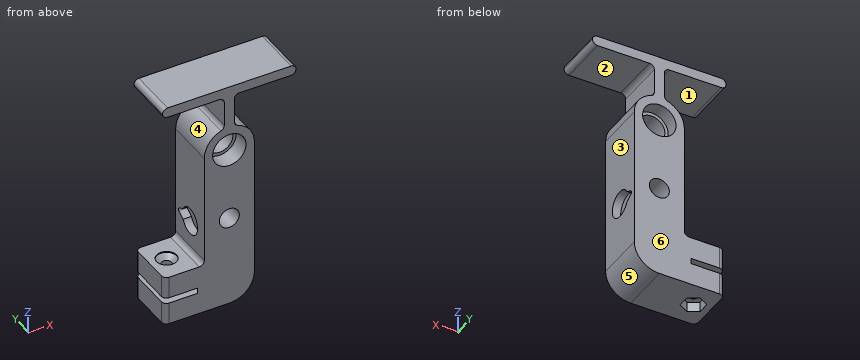
from build123d import *

# Parameters (mm, degrees)
SKETCH1_R           = 4
BOSS_EXTRUDE1_DEPTH = 7.5
SKETCH2_R           = 5
CUT_EXTRUDE1_DEPTH  = 4.1
SKETCH12_R          = 5
SKETCH12_R_2        = 4
CUT_EXTRUDE10_DEPTH = 1
CUT_EXTRUDE3_DEPTH  = 2.5
BOSS_EXTRUDE3_DEPTH = 15
CUT_EXTRUDE7_REACH  = 45.603
SKETCH7_W           = 10
SKETCH7_H           = 1.7
CUT_EXTRUDE8_REACH  = 76.732
SKETCH8_R           = 1.5
CUT_EXTRUDE9_DEPTH  = 3
CUT_EXTRUDE11_DEPTH = 1.7
BOSS_EXTRUDE2_START = -15
BOSS_EXTRUDE2_DEPTH = 15
FILLET8_R           = 1.5
CUT_EXTRUDE12_REACH = 45.829
SKETCH19_R          = 3


with BuildPart() as part:
    # Sketch1 → Boss-Extrude1 (new, symmetric)
    with BuildSketch(Plane(origin=(0, 0, 0), x_dir=(1, 0, 0), z_dir=(0, 1, 0))):
        with BuildLine():
            Line((7.5, 21), (-7.5, 21))
            Line((-7.5, 21), (-7.5, -13.499999984))
            ThreePointArc((-7.5, -13.499999984), (-8e-09, -21), (7.5, -13.5))
            Line((7.5, -13.5), (7.5, 21))
        make_face()
        with Locations(Location((0, -13.5, 0), (0, 0, 270))):
            Circle(SKETCH1_R, mode=Mode.SUBTRACT)
    extrude(amount=BOSS_EXTRUDE1_DEPTH, both=True)

    # Sketch2 → Cut-Extrude1 (cut)
    with BuildSketch(Plane(origin=(0, 7.5, 0), x_dir=(1, 0, 0), z_dir=(0, 1, 0))):
        with Locations(Location((0, -13.5, 0), (0, 0, 270))):
            Circle(SKETCH2_R)
    cut_extrude1 = extrude(amount=-CUT_EXTRUDE1_DEPTH, mode=Mode.SUBTRACT)

    # Mirror1: Cut-Extrude1 across plane
    add(cut_extrude1.mirror(Plane.ZX), mode=Mode.SUBTRACT)

    # Sketch12 → Cut-Extrude10 (cut)
    with BuildSketch(Plane.XZ.offset(3.4)):
        with Locations(Location((0, 13.5, 0), (0, 0, 90))):
            Circle(SKETCH12_R)
        with Locations(Location((0, 13.5, 0), (0, 0, 270))):
            Circle(SKETCH12_R_2, mode=Mode.SUBTRACT)
    extrude(amount=-CUT_EXTRUDE10_DEPTH, mode=Mode.SUBTRACT)

    # Sketch4 → Cut-Extrude3 (cut)
    with BuildSketch(Plane(origin=(7.5, 0, 0), x_dir=(0, 0, -1), z_dir=(1, 0, 0))):
        with BuildLine():
            Line((13.25, 3.596873642), (11.933012728, 5.87796251))
            ThreePointArc((11.933012728, 5.87796251), (11.500000041, 6.127962556), (11.066987313, 5.877962581))
            Line((11.066987313, 5.877962581), (9.75, 3.596873642))
            ThreePointArc((9.75, 3.596873642), (11.5, -4), (13.25, 3.596873642))
        make_face()
    cut_extrude3 = extrude(amount=-CUT_EXTRUDE3_DEPTH, mode=Mode.SUBTRACT)

    # Mirror2: Cut-Extrude3 across plane
    add(cut_extrude3.mirror(Plane(origin=(0, 0, 0), x_dir=(0, 0, 1), z_dir=(1, 0, 0))), mode=Mode.SUBTRACT)

    # Sketch18 → Boss-Extrude3 (add)
    with BuildSketch(Plane.XZ.offset(7.5)):
        with BuildLine():
            Line((-19.5, -21), (-19.5, -36))
            Line((-19.5, -36), (0, -36))
            ThreePointArc((0, -36), (5.303300859, -33.803300859), (7.5, -28.5))
            Line((7.5, -28.5), (7.5, -21))
            Line((7.5, -21), (-19.5, -21))
        make_face()
    extrude(amount=-BOSS_EXTRUDE3_DEPTH)

    # Sketch7 → Cut-Extrude7 (cut, up to next)
    with BuildSketch(Plane(origin=(0, 7.5, 0), x_dir=(1, 0, 0), z_dir=(0, 1, 0)), mode=Mode.PRIVATE) as cut_extrude7_sk1:
        with Locations((-14.5, 28.5)):
            Rectangle(SKETCH7_W, SKETCH7_H)
    cut_extrude7_tool1 = extrude(cut_extrude7_sk1.sketch, amount=-CUT_EXTRUDE7_REACH, mode=Mode.PRIVATE) & part.part
    add(cut_extrude7_tool1.solids().sort_by_distance((-14.5, 7.5, -28.5))[0], mode=Mode.SUBTRACT)

    # Cut-Extrude8: up to this face of the body (flat: up to its plane)
    cut_extrude8_end = Plane(part.part.faces().sort_by_distance((-13.5, 0, -21))[0])
    # Sketch8 → Cut-Extrude8 (cut, up to the picked face)
    with BuildSketch(Plane(origin=(-40.245190528, 0, -36), x_dir=(1, 0, 0), z_dir=(0, 0, 1)), mode=Mode.PRIVATE) as cut_extrude8_sk1:
        with Locations(Location((25.745190528, 0, 0), (0, 0, 180))):
            Circle(SKETCH8_R)
    cut_extrude8_tool1 = split(extrude(cut_extrude8_sk1.sketch, amount=CUT_EXTRUDE8_REACH, mode=Mode.PRIVATE), bisect_by=cut_extrude8_end, keep=Keep.BOTH, mode=Mode.PRIVATE)
    add(cut_extrude8_tool1.solids().sort_by(Axis((-14.5, 0, -36), (0, 0, 1)))[0], mode=Mode.SUBTRACT)

    # Sketch10 → CSK for M3 Flat Head Machine Screw1 (revolve, cut)
    with BuildSketch(Plane(origin=(-14.5, 0, -21), x_dir=(0, -1, 0), z_dir=(1, 0, 0))):
        Polygon((0, 0), (0, 5.901290929), (1.5, 5), (1.5, 1.8), (3, 0.3), (3, 0), align=None)
    revolve(axis=Axis((-14.5, 0, -14.65), (0, 0, -1)), mode=Mode.SUBTRACT)

    # Sketch11 → Cut-Extrude9 (cut)
    with BuildSketch(Plane(origin=(15, 0, -36), x_dir=(1, 0, 0), z_dir=(0, 0, 1))):
        Polygon((-29.5, -3.464101615), (-26.5, -1.732050808), (-26.5, 1.732050808), (-29.5, 3.464101615), (-32.5, 1.732050808), (-32.5, -1.732050808), align=None)
    extrude(amount=CUT_EXTRUDE9_DEPTH, mode=Mode.SUBTRACT)

    # Sketch13 → Cut-Extrude11 (cut)
    with BuildSketch(Plane(origin=(-44.653589838, 0, -29.35), x_dir=(1, 0, 0), z_dir=(0, 0, 1))):
        Polygon((35.153589838, 7.5), (42.653589838, 0), (35.153589838, -7.5), align=None)
    extrude(amount=CUT_EXTRUDE11_DEPTH, mode=Mode.SUBTRACT)

    # Sketch16 → Boss-Extrude2 (add)
    with BuildSketch(Plane.XZ.offset(7.5).offset(BOSS_EXTRUDE2_START)):
        with BuildLine():
            Line((1.5, 30.848469228), (-1.5, 30.848469228))
            Line((-1.5, 30.848469228), (-1.5, 20.848469228))
            ThreePointArc((-1.5, 20.848469228), (0, 21), (1.5, 20.848469228))
            Line((1.5, 20.848469228), (1.5, 30.848469228))
        make_face()
        Polygon((-20, 30.848469228), (-1.5, 30.848469228), (1.5, 30.848469228), (20, 30.848469228), (20, 33.848469228), (-20, 33.848469228), align=None)
    extrude(amount=BOSS_EXTRUDE2_DEPTH)

    # Fillet8
    fillet8_edges = [part.edges().sort_by_distance(p)[0] for p in [
        (20, 0, 30.848469228),
        (20, 0, 33.848469228),
        (-20, 0, 33.848469228),
        (-20, 0, 30.848469228),
        (-1.5, 0, 30.848469228),
        (-1.5, 0, 20.848469228),
        (1.5, 0, 20.848469228),
        (1.5, 0, 30.848469228),
        (-19.5, -7.5, -24.325),
        (-19.5, 7.5, -24.325),
        (-19.5, 7.5, -32.675),
        (-19.5, -7.5, -32.675),
        (-7.5, 0, -21),
    ]]
    fillet(fillet8_edges, radius=FILLET8_R - 0.0001)  # a hair under: the kernel refuses the full size

    # Sketch19 → Cut-Extrude12 (cut, up to next)
    with BuildSketch(Plane.XZ.offset(7.5), mode=Mode.PRIVATE) as cut_extrude12_sk1:
        with Locations(Location((0, -8.5, 0), (0, 0, 270))):
            Circle(SKETCH19_R)
    cut_extrude12_tool1 = extrude(cut_extrude12_sk1.sketch, amount=-CUT_EXTRUDE12_REACH, mode=Mode.PRIVATE) & part.part
    add(cut_extrude12_tool1.solids().sort_by_distance((0, -7.5, -8.5))[0], mode=Mode.SUBTRACT)


solid = part.part
Check sheet for the modelled part. Datum: model origin and axes. Units: mm. Face numbers are marked on the shaded views. A direction names the side the tool comes from. Round coordinates to 2 decimals unless told otherwise and drop trailing zeros. Write each loop counter-clockwise with the first axis right and the second up, starting at its lowest first coordinate (ties: lowest second). Pieces come first, ordered by that corner, then holes. Notation, with made-up numbers: (11, 76.25) - (64, 76.25) arc R17 cw to (64, 106.25) - close; hole circle Ø5 at (32, -13.5). An arc over 180 degrees is marked (long way). Return JSON: item names as keys, results as strings.
Q1. Scan lines: L1, parallel to Z at x = -12.5, y = 6.5; L2, parallel to Z at x = 4, y = -3.5; L3, parallel to Y at x = -14.5, z = -25.7. Record each from-to range of solid material in increasing order. Write a range as from..to.
Returned:
{"L1": "z = -36..-29.35, -27.65..-21, 30.85..33.85", "L2": "z = -34.84..10.5, 16.5..19.84, 30.85..33.85", "L3": "y = -7.5..-1.5, 1.5..7.5"}
Q2. Draft check along Z on the marked faces 4, 5 and 6. Enter one of: released by +Z, released by -Z, zero draft, split by the parting line, or undercut.
Returned:
{"face 4": "undercut", "face 5": "released by -Z", "face 6": "zero draft"}
Q3. Cross-section at C-C (x = 10). Record the boundary of the cut face in (y, z), then the cut area to 3 significant figures.
Returned:
{"outline": "(-7.5, 30.85) - (7.5, 30.85) - (7.5, 33.85) - (-7.5, 33.85) - close", "area": "45.0 mm²"}
Q4. Depth check by flat-ended pin: P1, Ø1.8, axis at x = -14, y = 1, coming from the -Z side; P2, Ø6.5, axis at y = 3, z = -11.5, coming from the +X side; P3, Ø8, axis at y = 2, z = 25, coming from the -X side. Enter the tip coordinate at first touch or a pass-through.
Returned:
{"P1": "stops at z = -33", "P2": "stops at x = 7.5", "P3": "stops at x = -1.87"}
Q5. Cross-section at B-B (z = -8.5). Record the boundary of the cut face in (x, y).
Returned:
{"outline": "(-7.5, -7.5) - (-3, -7.5) - (-3, 7.5) - (-7.5, 7.5) - (-7.5, 2.65) - (-5, 2.65) - (-5, -2.65) - (-7.5, -2.65) - close; (3, -7.5) - (7.5, -7.5) - (7.5, -2.65) - (5, -2.65) - (5, 2.65) - (7.5, 2.65) - (7.5, 7.5) - (3, 7.5) - close"}
Q6. Cross-section at A-A (z = 12.5). Record the boundary of the cut face in (x, y), then the cut area to 3 significant figures.
Returned:
{"outline": "(-7.5, -7.5) - (-4.9, -7.5) - (-4.9, -2.4) - (-3.87, -2.4) - (-3.87, 3.4) - (-4.9, 3.4) - (-4.9, 7.5) - (-7.5, 7.5) - close; (3.87, -2.4) - (4.9, -2.4) - (4.9, -7.5) - (7.5, -7.5) - (7.5, 7.5) - (4.9, 7.5) - (4.9, 3.4) - (3.87, 3.4) - close", "area": "89.9 mm²"}
Q7. Access from +Z, -Z, +X, -X, +Y, -Y to the whole of each face (thin tool, end or side, straight path). Record for the marked faces 1, 2 and 3.
Returned:
{"face 1": "-X, +Y, -Y", "face 2": "+X, +Y, -Y", "face 3": "-Z, +X, +Y, -Y"}
